from build123d import *

# Parameters (mm, degrees)
BOSS_EXTRUDE1_DEPTH  = 76.2
CUT_EXTRUDE1_START   = -36.5125
CUT_EXTRUDE1_DEPTH   = 73.025
M5_CLEARANCE_HOLE1_D = 5.5
CUT_EXTRUDE2_REACH   = 145.772
SKETCH10_R           = 19.05


with BuildPart() as part:
    # Sketch1 → Boss-Extrude1 (new body)
    with BuildSketch(Plane.XY):
        Polygon((36.5125, -121.15027858), (36.5125, -66.416505111), (0, -3.175), (-36.5125, -66.416505111), (-36.5125, -121.15027858), align=None)
    extrude(amount=BOSS_EXTRUDE1_DEPTH)

    # Sketch2 → Cut-Extrude1 (cut)
    with BuildSketch(Plane(origin=(0, 0, 0), x_dir=(0, 0, -1), z_dir=(1, 0, 0)).offset(CUT_EXTRUDE1_START)):
        with BuildLine():
            Line((-76.2, -121.15027858), (0, -121.15027858))
            ThreePointArc((0, -121.15027858), (-23.393988511, -62.928903921), (-68.2625, -19.067487592))
            Line((-68.2625, -19.067487592), (-68.2625, -3.175))
            Line((-68.2625, -3.175), (-76.2, -3.175))
            Line((-76.2, -3.175), (-76.2, -22.225))
            Line((-76.2, -22.225), (-76.2, -66.416505111))
            Line((-76.2, -66.416505111), (-76.2, -121.15027858))
        make_face()
    extrude(amount=CUT_EXTRUDE1_DEPTH, mode=Mode.SUBTRACT)

    # M5 Clearance Hole1 (through all)
    with Locations(Plane(origin=(0, 0, 0), x_dir=(-1, 0, 0), z_dir=(0, 0, -1))):
        with Locations((-15.875, -81.009177721), (15.875, -81.009177721), (0, -38.1)):
            Hole(M5_CLEARANCE_HOLE1_D / 2)

    # Sketch10 → Cut-Extrude2 (cut, up to next)
    with BuildSketch(Plane(origin=(0, 0, 0), x_dir=(-1, 0, 0), z_dir=(0, 0, -1)), mode=Mode.PRIVATE) as cut_extrude2_sk1:
        Circle(SKETCH10_R)
    cut_extrude2_tool1 = extrude(cut_extrude2_sk1.sketch, amount=-CUT_EXTRUDE2_REACH, mode=Mode.PRIVATE) & part.part
    add(cut_extrude2_tool1.solids().sort_by_distance((0, 0, 0))[0], mode=Mode.SUBTRACT)


solid = part.part
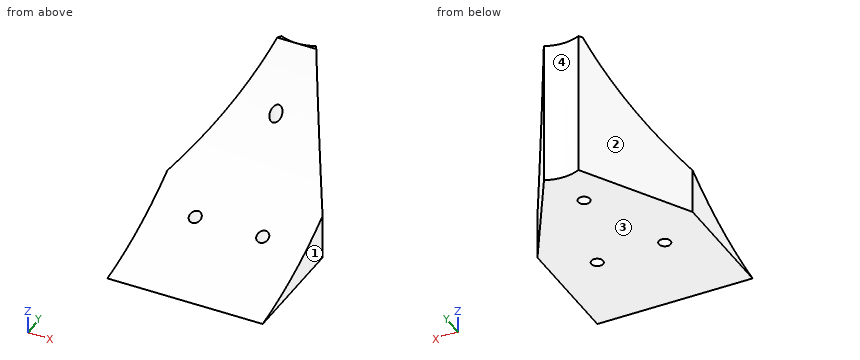
Check sheet for the modelled part. Datum: model origin and axes. Units: mm. Face numbers are marked on the shaded views. Coordinates: 2 decimals unless noted, no trailing zeros. Loops run counter-clockwise (first coordinate to the right, second up) from the corner with the lowest first, then second, coordinate; pieces in that order, holes last. Notation, with made-up numbers: (-15, 19.25) -> (8, 19.25) arc R36 cw to (8, 56.25) -> close; hole circle Ø3 at (-24.5, 43.5). An arc over 180 degrees is marked (long way). Answer in a Markdown table with one row per item.
1. Go/stop test with flat-tipped pins: pin 1 (3.5 mm diameter, centred on x = -15.88, y = -81.01, fed in from -Z); pin 2 (6 mm diameter, centred on x = 6.5, z = 10, fed in from +Y); pin 3 (10 mm diameter, centred on x = -18.5, z = 22.5, fed in from +Y); pin 4 (12 mm diameter, centred on x = -2, y = -91, fed in from +Z). Record where each tip stops, or that it passes through.
Check values:
| item | result |
|---|---|
| pin 1 | passes through |
| pin 2 | stops at y = -17.23 |
| pin 3 | stops at y = -26.56 |
| pin 4 | stops at z = 11.15 |
2. Sectioned sample at D-D, the plane z = 23.5. Record the boundary of the cut face in (x, y).
Check values:
| item | result |
|---|---|
| outline | (-34.41, -62.77) -> (34.41, -62.77) -> (8.12, -17.23) arc R19.05 cw to (-8.12, -17.23) -> close; hole circle Ø5.5 at (0, -38.1) |
3. Sectioned sample at A-A, the plane z = 16. Record the boundary of the cut face in (x, y).
Check values:
| item | result |
|---|---|
| outline | (-36.51, -75.2) -> (36.51, -75.2) -> (36.51, -66.42) -> (8.12, -17.23) arc R19.05 cw to (-8.12, -17.23) -> (-36.51, -66.42) -> close; hole circle Ø5.5 at (0, -38.1) |
4. Material ranges on line 1 along Z through (x, y) = (-0.5, -46); line 2 along Y through (x, z) = (0, 36.5); line 3 along Y through (x, z) = (-0.5, 40.5), recorded low to high. Write a range as [from, to].
Check values:
| item | result |
|---|---|
| line 1 | z = [0, 36.53] |
| line 2 | y = [-46.03, -40.85], [-35.35, -19.05] |
| line 3 | y = [-41.73, -40.8], [-35.4, -19.04] |
5. Release check for a two-part mould opening along X. For the marked faces 1, 2, 3 and 4 record: released by +X, released by -X, zero draft, split by the parting line, or undercut.
Check values:
| item | result |
|---|---|
| face 1 | released by +X |
| face 2 | released by -X |
| face 3 | zero draft |
| face 4 | undercut |
6. Sectioned sample at C-C, the plane y = -38.1. Record the boundary of the cut face in (x, z).
Check values:
| item | result |
|---|---|
| outline | (-20.16, 0) -> (-2.75, 0) -> (-2.75, 44.13) -> (-20.16, 44.13) -> close; (2.75, 0) -> (20.16, 0) -> (20.16, 44.13) -> (2.75, 44.13) -> close |
